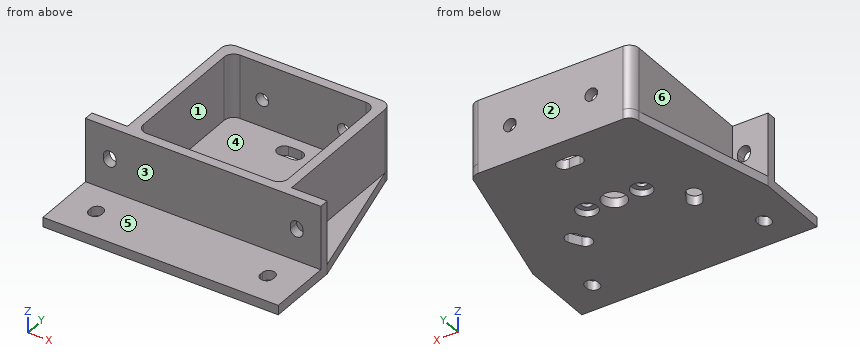
from build123d import *

# Parameters (mm, degrees)
SKETCH1_W           = 74
SKETCH1_H           = 70
SKETCH1_R           = 3.75
SKETCH1_R_2         = 1.625
BOSS_EXTRUDE1_DEPTH = 3
BOSS_EXTRUDE2_DEPTH = 20
CUT_EXTRUDE2_DEPTH  = 3
FILLET1_R           = 3
FILLET2_R           = 3
FILLET4_R           = 3
FILLET5_R           = 3
CUT_EXTRUDE4_DEPTH  = 3
FILLET6_R           = 3
FILLET7_R           = 3
FILLET8_R           = 3
FILLET9_R           = 3
SKETCH11_R          = 2
CUT_EXTRUDE5_DEPTH  = 3
SKETCH12_R          = 3.25
CUT_EXTRUDE6_DEPTH  = 2


with BuildPart() as part:
    # Sketch1 → Boss-Extrude1 (new body)
    with BuildSketch(Plane.XY):
        with Locations((37, 35)):
            Rectangle(SKETCH1_W, SKETCH1_H)
        with Locations((37, 40)):
            Circle(SKETCH1_R, mode=Mode.SUBTRACT)
        with Locations((28.4, 40)):
            Circle(SKETCH1_R_2, mode=Mode.SUBTRACT)
        with Locations((45.6, 40)):
            Circle(SKETCH1_R_2, mode=Mode.SUBTRACT)
        with BuildLine():
            Line((8, 10.5), (8, 9.5))
            ThreePointArc((8, 9.5), (10, 7.5), (12, 9.5))
            Line((12, 9.5), (12, 10.5))
            ThreePointArc((12, 10.5), (10, 12.5), (8, 10.5))
        make_face(mode=Mode.SUBTRACT)
        with BuildLine():
            Line((66, 10.5), (66, 9.5))
            ThreePointArc((66, 9.5), (64, 7.5), (62, 9.5))
            Line((62, 9.5), (62, 10.5))
            ThreePointArc((62, 10.5), (64, 12.5), (66, 10.5))
        make_face(mode=Mode.SUBTRACT)
        with BuildLine():
            ThreePointArc((34.973628981, 63.161526731), (32.928291332, 60.723988239), (35.365829823, 58.678650589))
            ThreePointArc((35.365829823, 58.678650589), (37, 58.75), (38.634170177, 58.678650589))
            ThreePointArc((38.634170177, 58.678650589), (41.071708668, 60.723988239), (39.026371019, 63.161526731))
            ThreePointArc((39.026371019, 63.161526731), (37, 63.25), (34.973628981, 63.161526731))
        make_face(mode=Mode.SUBTRACT)
        with BuildLine():
            ThreePointArc((15.928343951, 30.174125415), (17.016645383, 33.164209024), (20.006728993, 32.075907592))
            ThreePointArc((20.006728993, 32.075907592), (20.762023679, 30.625), (21.64089917, 29.245441818))
            ThreePointArc((21.64089917, 29.245441818), (21.088354052, 26.111802737), (17.95471497, 26.664347855))
            ThreePointArc((17.95471497, 26.664347855), (16.864909362, 28.375), (15.928343951, 30.174125415))
        make_face(mode=Mode.SUBTRACT)
        with BuildLine():
            ThreePointArc((58.071656049, 30.174125415), (56.983354617, 33.164209024), (53.993271007, 32.075907592))
            ThreePointArc((53.993271007, 32.075907592), (53.237976321, 30.625), (52.35910083, 29.245441818))
            ThreePointArc((52.35910083, 29.245441818), (52.911645948, 26.111802737), (56.04528503, 26.664347855))
            ThreePointArc((56.04528503, 26.664347855), (57.135090638, 28.375), (58.071656049, 30.174125415))
        make_face(mode=Mode.SUBTRACT)
    extrude(amount=BOSS_EXTRUDE1_DEPTH)

    # Sketch2 → Loft1 section 0
    with BuildSketch(Plane.XY.offset(3)):
        with BuildLine():
            Line((0, 23), (74, 23))
            Line((74, 23), (74, 20))
            Line((74, 20), (0, 20))
            Line((0, 20), (0, 23))
        make_face()
    # Sketch3 → Loft1 section 1
    with BuildSketch(Plane.XY.offset(23)):
        with BuildLine():
            Line((0, 23), (74, 23))
            Line((74, 23), (74, 20))
            Line((74, 20), (0, 20))
            Line((0, 20), (0, 23))
        make_face()
    loft()

    # Sketch4 → Boss-Extrude2 (add)
    with BuildSketch(Plane.XY.offset(3)):
        Polygon((14.2, 23), (14.2, 67), (59.8, 67), (59.8, 23), (62.8, 23), (62.8, 70), (11.2, 70), (11.2, 23), align=None)
    extrude(amount=BOSS_EXTRUDE2_DEPTH)

    # Sketch8 → Cut-Extrude2 (cut)
    with BuildSketch(Plane(origin=(0, 23, 0), x_dir=(1, 0, 0), z_dir=(0, 1, 0))):
        with BuildLine():
            Line((5.6, -12.5), (5.6, -13.5))
            ThreePointArc((5.6, -13.5), (7.6, -15.5), (9.6, -13.5))
            Line((9.6, -13.5), (9.6, -12.5))
            ThreePointArc((9.6, -12.5), (7.6, -10.5), (5.6, -12.5))
        make_face()
        with BuildLine():
            Line((68.4, -12.5), (68.4, -13.5))
            ThreePointArc((68.4, -13.5), (66.4, -15.5), (64.4, -13.5))
            Line((64.4, -13.5), (64.4, -12.5))
            ThreePointArc((64.4, -12.5), (66.4, -10.5), (68.4, -12.5))
        make_face()
    extrude(amount=-CUT_EXTRUDE2_DEPTH, mode=Mode.SUBTRACT)

    # Fillet1
    fillet1_edges = [part.edges().sort_by_distance(p)[0] for p in [
        (11.2, 70, 13),
    ]]
    fillet(fillet1_edges, radius=FILLET1_R)

    # Fillet2
    fillet2_edges = [part.edges().sort_by_distance(p)[0] for p in [
        (62.8, 70, 13),
    ]]
    fillet(fillet2_edges, radius=FILLET2_R)

    # Fillet4
    fillet4_edges = [part.edges().sort_by_distance(p)[0] for p in [
        (59.8, 67, 13),
    ]]
    fillet(fillet4_edges, radius=FILLET4_R)

    # Fillet5
    fillet5_edges = [part.edges().sort_by_distance(p)[0] for p in [
        (14.2, 67, 13),
    ]]
    fillet(fillet5_edges, radius=FILLET5_R)

    # Sketch10 → Cut-Extrude4 (cut)
    with BuildSketch(Plane.XY.offset(3)):
        Polygon((0, 23), (11.2, 67), (11.2, 70), (0, 70), align=None)
        Polygon((74, 23), (62.8, 67), (62.8, 70), (74, 70), align=None)
    extrude(amount=-CUT_EXTRUDE4_DEPTH, mode=Mode.SUBTRACT)

    # Fillet6
    fillet6_edges = [part.edges().sort_by_distance(p)[0] for p in [
        (62.8, 70, 1.5),
    ]]
    fillet(fillet6_edges, radius=FILLET6_R - 0.0001)  # a hair under: the kernel refuses the full size

    # Fillet7
    fillet7_edges = [part.edges().sort_by_distance(p)[0] for p in [
        (11.2, 70, 1.5),
    ]]
    fillet(fillet7_edges, radius=FILLET7_R - 0.0001)  # a hair under: the kernel refuses the full size

    # Fillet8
    fillet8_edges = [part.edges().sort_by_distance(p)[0] for p in [
        (14.2, 23, 13),
    ]]
    fillet(fillet8_edges, radius=FILLET8_R)

    # Fillet9
    fillet9_edges = [part.edges().sort_by_distance(p)[0] for p in [
        (59.8, 23, 13),
    ]]
    fillet(fillet9_edges, radius=FILLET9_R)

    # Sketch11 → Cut-Extrude5 (cut)
    with BuildSketch(Plane(origin=(0, 70, 0), x_dir=(1, 0, 0), z_dir=(0, 1, 0))):
        with Locations(Location((24.2, -11.5, 0), (0, 0, 270))):
            Circle(SKETCH11_R)
        with Locations(Location((49.8, -11.5, 0), (0, 0, 90))):
            Circle(SKETCH11_R)
    extrude(amount=-CUT_EXTRUDE5_DEPTH, mode=Mode.SUBTRACT)

    # Sketch12 → Cut-Extrude6 (cut)
    with BuildSketch(Plane(origin=(0, 0, 0), x_dir=(-1, 0, 0), z_dir=(0, 0, -1))):
        with Locations((-45.6, 40)):
            Circle(SKETCH12_R)
        with Locations((-28.4, 40)):
            Circle(SKETCH12_R)
    extrude(amount=-CUT_EXTRUDE6_DEPTH, mode=Mode.SUBTRACT)


solid = part.part
CAD build for the part. Positions are in the model's coordinates, mm. Face numbers are marked on the shaded views. A direction names the side the tool comes from. Round coordinates to 2 decimals unless told otherwise and drop trailing zeros. Write each loop counter-clockwise with the first axis right and the second up, starting at its lowest first coordinate (ties: lowest second). Pieces come first, ordered by that corner, then holes. Notation, with made-up numbers: M 16.25,-11 L 52.25,-11 A7 ccw 52.25,2 Z; hole C -11.75,66 d2. An arc over 180 degrees is marked long. Put each result on its own line as item: value. Start each with the question number.
1) Saw through at C-C, the plane z = 11.5. Count the separate pieces of the cut face and the enclosed holes in it, and give its area (3 significant figures).
2) Saw through at A-A, the plane x = 37. Write the cut outline in (y, z).
3) Pin check, flat tips, straight feed: pin 1 Ø12.5 at (x, z) = (6, 16.5) entering from +Y; pin 2 Ø10 at (x, z) = (63.5, 8) entering from +Y; pin 3 Ø16 at (x, y) = (25.5, 8.5) entering from +Z; pin 4 Ø5 at (x, y) = (28.4, 40) entering from -Z. Stop position of each tip, or through.
4) Saw through at D-D, the plane y = 5. Write the cut outline in (x, z).
5) Saw through at B-B, the plane x = 24.2. Write the cut outline in (y, z), and give its area (3 significant figures).
6) Drill centre lines: probe 1 along X at (y, z) = (58.5, 12.5); probe 2 along Y at (x, z) = (42, 8); probe 3 along Y at (x, z) = (37, 2). Where is each one in solid material? Low to high. Write a range as [from, to].
7) Pull direction Y, two halves, no side cores. Call the marked faces 1, 2 and 3: pulls with the +Y half, pulls with the -Y half, needs draft (parallel to the pull), parting line crosses it, or undercut.
8) 3-axis set-ups, long thin cutter, end or side, ignore diameter. For the marked faces 4, 5 and 6: which of +Z, -Z, +X, -X, +Y, -Y reach the whole face in a straight line?
Resolved:
1. separate pieces: 4
1. enclosed holes: 0
1. area: 600 mm²
2. outline: M 0,0 L 36.25,0 L 36.25,3 L 23,3 L 23,23 L 20,23 L 20,3 L 0,3 Z; M 43.75,0 L 58.75,0 L 58.75,3 L 43.75,3 Z; M 63.25,0 L 70,0 L 70,23 L 67,23 L 67,3 L 63.25,3 Z
3. pin 1: y = 69.28
3. pin 2: y = 70
3. pin 3: z = 3
3. pin 4: z = 2
4. outline: M 0,0 L 74,0 L 74,3 L 0,3 Z
5. outline: M 0,0 L 70,0 L 70,9.5 L 67,9.5 L 67,3 L 23,3 L 23,23 L 20,23 L 20,3 L 0,3 Z; M 67,13.5 L 70,13.5 L 70,23 L 67,23 Z
5. area: 318 mm²
6. probe 1: [11.2, 14.2], [59.8, 62.8]
6. probe 2: [20, 23], [67, 70]
6. probe 3: [0, 36.25], [43.75, 58.75], [63.25, 70]
7. face 1: undercut
7. face 2: pulls with the +Y half
7. face 3: pulls with the -Y half
8. face 4: +Z
8. face 5: +Z, +X, -X, -Y
8. face 6: +Z, -X, +Y
